Study the drawing (mm; zero at the part's minimum x, y, z) and answer. Coordinates: 2 decimals unless noted, no trailing zeros. Order: outer loops, then holes, each group sorted by start corner. A loop starts at its lowest first (then second) coordinate and runs counter-clockwise, first axis right, second up.
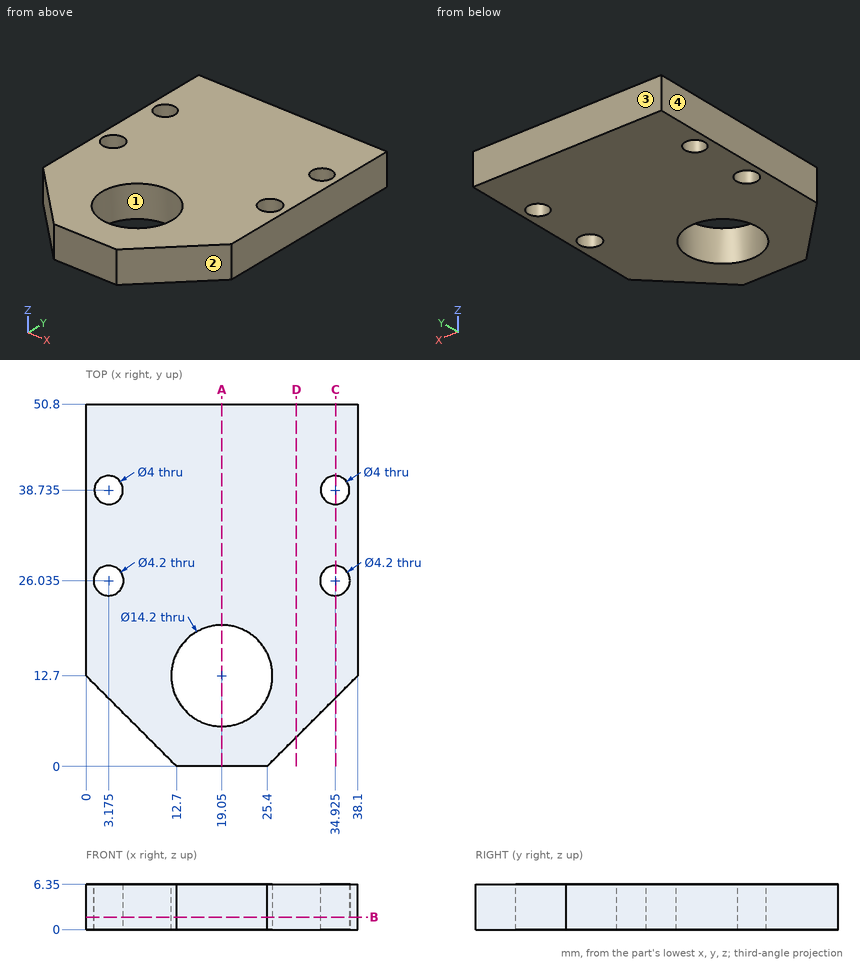
1) A cutting plane is placed at A-A, the plane x = 19.05. Determine the outline of the cut face in (y, z), and give its area (3 significant figures).
A:
outline: (0, 0) - (5.6, 0) - (5.6, 6.35) - (0, 6.35) - close; (19.8, 0) - (50.8, 0) - (50.8, 6.35) - (19.8, 6.35) - close
area: 232 mm2
2) A cutting plane is placed at D-D, the plane x = 29.5. Determine the outline of the cut face in (y, z), and give its area (3 significant figures).
A:
outline: (4.1, 0) - (50.8, 0) - (50.8, 6.35) - (4.1, 6.35) - close
area: 297 mm2
3) A cutting plane is placed at C-C, the plane x = 35. Determine the outline of the cut face in (y, z).
A:
outline: (9.6, 0) - (23.94, 0) - (23.94, 6.35) - (9.6, 6.35) - close; (28.13, 0) - (36.74, 0) - (36.74, 6.35) - (28.13, 6.35) - close; (40.73, 0) - (50.8, 0) - (50.8, 6.35) - (40.73, 6.35) - close
4) A flat-ended cylindrical pin translates along its axis: pin 1 Ø1.5 at (x, z) = (32.5, 1) entering from -Y. Find the tip coordinate at first contact, or state that the pin passes through.
A:
pin 1: stops at y = 6.35
5) A cutting plane is placed at B-B, the plane z = 1.75. Determine the outline of the cut face in (x, y) (3 decimals).
A:
outline: (0, 12.7) - (12.7, 0) - (25.4, 0) - (38.1, 12.7) - (38.1, 50.8) - (0, 50.8) - close; hole circle Ø4.2 at (3.175, 26.035); hole circle Ø4 at (3.175, 38.735); hole circle Ø14.2 at (19.05, 12.7); hole circle Ø4.2 at (34.925, 26.035); hole circle Ø4 at (34.925, 38.735)
6) Determine the mould class of the marked faces 1, 2, 3 and 4 for opening direction Y: pulls with the +Y half, pulls with the -Y half, needs draft (parallel to the pull), parting line crosses it, or undercut.
A:
face 1: undercut
face 2: pulls with the -Y half
face 3: pulls with the +Y half
face 4: needs draft
7) Straight lines are drawn through the part: line 1 (Y direction, x = 3, z = 5); line 2 (Y direction, x = 19.05, z = 1.5); line 3 (X direction, y = 24.5, z = 5). For each, find the intervals that lie inside material, in ascending order.
A:
line 1: y = 9.7 to 23.94, 28.13 to 36.74, 40.73 to 50.8
line 2: y = 0 to 5.6, 19.8 to 50.8
line 3: x = 0 to 1.74, 4.61 to 33.49, 36.36 to 38.1
